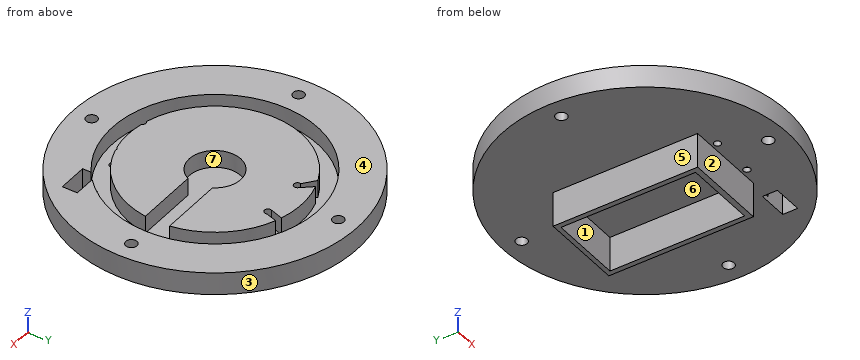
from build123d import *

# Parameters (mm, degrees)
F0_R      = 57.15
F1_DEPTH  = 9
F2_R      = 41.1777557501
F2_R_2    = 34.7361553424
F3_DEPTH  = 7
F5_DEPTH  = 7
F6_W      = 12
F6_H      = 6
F7_DEPTH  = 9
F9_D      = 4.4958
F10_W     = 33
F10_H     = 58
F10_W_2   = 29
F10_H_2   = 54
F11_DEPTH = 14
F13_D     = 2.794
F15_DEPTH = 7


with BuildPart() as f1:
    # F0 (on Top) → F1 (new body)
    with BuildSketch(Plane.XY):
        Circle(F0_R)
    extrude(amount=F1_DEPTH)

    # F2 (on face) → F3 (cut)
    with BuildSketch(Plane.XY.offset(9)):
        Circle(F2_R)
        Circle(F2_R_2, mode=Mode.SUBTRACT)
    extrude(amount=-F3_DEPTH, mode=Mode.SUBTRACT)

    # F4 (on face) → F5 (cut)
    with BuildSketch(Plane.XY.offset(9)):
        with BuildLine():
            ThreePointArc((9.2364512329, -4.5815780759), (10.0382703258, -2.3528743932), (10.3103292403, 0))
            ThreePointArc((10.3103292403, 0), (9.9709085428, 2.6237133751), (8.9749942157, 5.0746790905))
            Line((8.9749942157, 5.0746790905), (8.9749942157, -4.5815780759))
            Line((8.9749942157, -4.5815780759), (9.2364512329, -4.5815780759))
        make_face()
        with BuildLine():
            Line((37.7700850368, 5.0746790905), (34.3634707226, 5.0746790905))
            ThreePointArc((34.3634707226, 5.0746790905), (34.6428588969, 2.544172837), (34.7361553424, 0))
            ThreePointArc((34.7361553424, 0), (34.6602041198, -2.2958088649), (34.4326825895, -4.5815780759))
            Line((34.4326825895, -4.5815780759), (37.7700850368, -4.5815780759))
            Line((37.7700850368, -4.5815780759), (37.7700850368, 5.0746790905))
        make_face()
        with BuildLine():
            Line((8.9749942157, -4.5815780759), (8.9749942157, 5.0746790905))
            ThreePointArc((8.9749942157, 5.0746790905), (-10.3065518942, -0.27906468), (9.2364512329, -4.5815780759))
            Line((9.2364512329, -4.5815780759), (8.9749942157, -4.5815780759))
        make_face()
        with BuildLine():
            ThreePointArc((8.9749942157, 5.0746790905), (9.9709085428, 2.6237133751), (10.3103292403, 0))
            ThreePointArc((10.3103292403, 0), (10.0382703258, -2.3528743932), (9.2364512329, -4.5815780759))
            Line((9.2364512329, -4.5815780759), (34.4326825895, -4.5815780759))
            ThreePointArc((34.4326825895, -4.5815780759), (34.6602041198, -2.2958088649), (34.7361553424, 0))
            ThreePointArc((34.7361553424, 0), (34.6428588969, 2.544172837), (34.3634707226, 5.0746790905))
            Line((34.3634707226, 5.0746790905), (8.9749942157, 5.0746790905))
        make_face()
    extrude(amount=-F5_DEPTH, mode=Mode.SUBTRACT)

    # F6 (on face) → F7 (cut)
    with BuildSketch(Plane(origin=(0, 0, 0), x_dir=(1, 0, 0), z_dir=(0, 0, -1))):
        with Locations((30.4291332662, 33.5408807993)):
            Rectangle(F6_W, F6_H)
    extrude(amount=-F7_DEPTH, mode=Mode.SUBTRACT)

    # F9 (through all)
    with Locations(Plane.XY.offset(9)):
        with Locations((0, 49.4705886591), (-49.4705886591, 0), (0, -49.4705886591), (49.4705886591, 0)):
            Hole(F9_D / 2)

    # F10 (on face) → F11 (join)
    with BuildSketch(Plane(origin=(0, 0, 0), x_dir=(1, 0, 0), z_dir=(0, 0, -1))):
        with Locations((0.185111627, 3.1867184639)):
            Rectangle(F10_W, F10_H)
        with Locations((0.1965364888, 2.9830217808)):
            Rectangle(F10_W_2, F10_H_2, mode=Mode.SUBTRACT)
    extrude(amount=F11_DEPTH)

    # F13 (through all)
    with Locations(Plane(origin=(0, 0, 0), x_dir=(1, 0, 0), z_dir=(0, 0, -1))):
        with Locations((-8.0456975847, 34.5294550061), (9.3866474926, 34.5294550061), (-8.0456975847, -27.6012141258), (9.3866474926, -27.6012141258)):
            Hole(F13_D / 2)

    # F14 (on face) → F15 (cut)
    with BuildSketch(Plane.XY.offset(9)):
        with BuildLine():
            Line((-14.0573482538, 31.7646257344), (-9.3722739345, 28.0391686762))
            ThreePointArc((-9.3722739345, 28.0391686762), (-8.3136402911, 28.9722778391), (-6.9816011946, 28.5063703953))
            Line((-6.9816011946, 28.5063703953), (-10.8128362283, 33.0103477817))
            ThreePointArc((-10.8128362283, 33.0103477817), (-12.4506817042, 32.4280898771), (-14.0573482538, 31.7646257344))
        make_face()
        with BuildLine():
            ThreePointArc((12.1452810093, 32.5437034951), (10.9819164525, 32.9544837466), (9.804697926, 33.3236910704))
            Line((9.804697926, 33.3236910704), (8.0600711429, 28.0391686762))
            ThreePointArc((8.0600711429, 28.0391686762), (9.3866474926, 28.9982141258), (10.7132238424, 28.0391686762))
            Line((10.7132238424, 28.0391686762), (12.1452810093, 32.5437034951))
        make_face()
    extrude(amount=-F15_DEPTH, mode=Mode.SUBTRACT)


solid = f1.part
Check sheet for the modelled part. Datum: model origin and axes. Units: mm. Face numbers are marked on the shaded views. A direction names the side the tool comes from. Round coordinates to 2 decimals unless told otherwise and drop trailing zeros. Write each loop counter-clockwise with the first axis right and the second up, starting at its lowest first coordinate (ties: lowest second). Pieces come first, ordered by that corner, then holes. Notation, with made-up numbers: (1.25, 4) -> (59.25, 4) arc R31 cw to (59.25, 32) -> close; hole circle Ø2 at (72.5, 34). An arc over 180 degrees is marked (long way). Answer as CSV lines item,"result". Start each with the question number.
1) Material ranges on line 1 (X direction, y = -2.5, z = -10); line 2 (Y direction, x = -7.5, z = -3.5); line 3 (Y direction, x = 17, z = 7), recorded low to high. Write a range as from..to.
2) Section check C-C on x = 0. State how many separate pieces and enclosed holes the cut face has, and give its area (3 significant figures).
3) Release check for a two-part mould opening along Y. For the marked faces 1, 2, 3 and 4 record: pulls with the +Y half, pulls with the -Y half, needs draft (parallel to the pull), parting line crosses it, or undercut.
4) Section check A-A on z = 6. Enter the section's corners in (x, y) (3 decimals).
5) Section check B-B on y = 0. Enter the section's corners in (x, z), and give its area (3 significant figures).
6) Go/stop test with flat-tipped pins: P1, Ø7, axis at x = 29.5, z = 3, coming from the +Y side; P2, Ø3, axis at x = 4, y = 15.5, coming from the -Z side; P3, Ø4, axis at x = -10, z = -7.5, coming from the +Y side; P4, Ø2.5, axis at x = 49.47, y = 0, coming from the -Z side. Record where each tip stops, or that it passes through.
7) Section check D-D on z = -4. Enter the section's corners in (x, y).
8) Tool access check on the marked faces 5, 6 and 7. Record the directions out of +Z, -Z, +X, -X, +Y, -Y that give a thin tool (end or side, any length) a straight path to the whole face; none if there is none.
Found:
1,line 1,"x = -16.31..-14.3, 14.7..16.69"
1,line 2,"y = -32.19..-29.98, 24.02..25.81"
1,line 3,"y = -54.56..-37.5, -30.29..-4.58, 5.07..30.29, 37.5..54.56"
2,separate pieces,"3"
2,enclosed holes,"0"
2,area,"769 mm^2"
3,face 1,"undercut"
3,face 2,"pulls with the -Y half"
3,face 3,"parting line crosses it"
3,face 4,"needs draft"
4,outline,"circle Ø114.3 at (0, 0); (-14.057, 31.765) arc R34.736 ccw to (-9.033, -33.541) arc R1.397 cw to (-6.723, -34.079) arc R34.736 ccw to (8.229, -33.747) arc R1.397 cw to (9.989, -33.269) arc R34.736 ccw to (34.433, -4.582) -> (9.236, -4.582) arc R10.31 cw (long way) to (8.975, 5.075) -> (34.363, 5.075) arc R34.736 ccw to (12.145, 32.544) -> (10.713, 28.039) arc R1.397 cw (long way) to (8.06, 28.039) -> (9.805, 33.324) arc R34.736 ccw to (-10.813, 33.01) -> (-6.982, 28.506) arc R1.397 cw (long way) to (-9.372, 28.039) -> close; hole circle Ø4.496 at (-49.471, 0); hole circle Ø4.496 at (0, -49.471); hole circle Ø4.496 at (0, 49.471); hole (24.429, -36.541) -> (36.429, -36.541) -> (36.429, -30.541) -> (27.62, -30.541) arc R41.178 ccw (long way) to (24.429, -33.149) -> close; hole circle Ø4.496 at (49.471, 0)"
5,outline,"(-57.15, 0) -> (-51.72, 0) -> (-51.72, 9) -> (-57.15, 9) -> close; (-47.22, 0) -> (-16.31, 0) -> (-16.31, -14) -> (-14.3, -14) -> (-14.3, 0) -> (14.7, 0) -> (14.7, -14) -> (16.69, -14) -> (16.69, 0) -> (47.22, 0) -> (47.22, 9) -> (41.18, 9) -> (41.18, 2) -> (-10.31, 2) -> (-10.31, 9) -> (-34.74, 9) -> (-34.74, 2) -> (-41.18, 2) -> (-41.18, 9) -> (-47.22, 9) -> close; (51.72, 0) -> (57.15, 0) -> (57.15, 9) -> (51.72, 9) -> close"
5,area,"598 mm^2"
6,P1,"stops at y = 50.89"
6,P2,"stops at z = 0"
6,P3,"stops at y = 25.81"
6,P4,"passes through"
7,outline,"(-16.31, -32.19) -> (16.69, -32.19) -> (16.69, 25.81) -> (-16.31, 25.81) -> close; hole (-14.3, -29.98) -> (14.7, -29.98) -> (14.7, 24.02) -> (-14.3, 24.02) -> close"
8,face 5,"-Z, -X, +Y, -Y"
8,face 6,"-Z"
8,face 7,"+Z"
